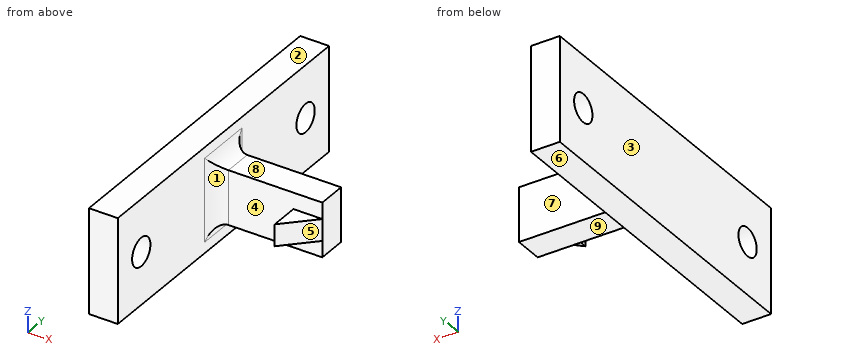
```python
from build123d import *

# Parameters (mm, degrees)
BOSS_EXTRUDE1_DEPTH      = 1
BOSS_EXTRUDE1_DEPTH_BACK = 1
SKETCH2_R                = 2
SKETCH2_R_2              = 1
BOSS_EXTRUDE2_DEPTH      = 4
SKETCH4_R                = 1.07
CUT_EXTRUDE1_DEPTH       = 233.583689314
BOSS_EXTRUDE3_DEPTH      = 2
SKETCH8_W                = 4
SKETCH8_H                = 8
BOSS_EXTRUDE4_DEPTH      = 2
CUT_EXTRUDE2_DEPTH       = 2
SKETCH10_W               = 16.5
SKETCH10_H               = 4
BOSS_EXTRUDE5_DEPTH      = 2.75
SKETCH11_W               = 16.5
SKETCH11_H               = 4
BOSS_EXTRUDE6_DEPTH      = 2.75
BOSS_EXTRUDE7_DEPTH      = 0.5
BOSS_EXTRUDE8_DEPTH      = 0.5
SKETCH14_W               = 1.779922348
SKETCH14_H               = 4
BOSS_EXTRUDE9_DEPTH      = 7.5
CUT_EXTRUDE3_DEPTH       = 10
CUT_EXTRUDE3_DEPTH_BACK  = 2
SKETCH15_W               = 40
SKETCH15_H               = 27.31360861
SKETCH16_W               = 14.5
SKETCH16_H               = 45
BOSS_EXTRUDE10_DEPTH     = 4
SKETCH18_R               = 1.95
CUT_EXTRUDE4_DEPTH       = 4
FILLET1_R                = 2


with BuildPart() as part:
    # Sketch2 → Boss-Extrude1 (new, two sides: drawn at the far end of the back side and taken through both)
    # profile 1 of 2: a face of its own
    with BuildSketch(Plane.XY.offset(-2.5).offset(-BOSS_EXTRUDE1_DEPTH_BACK)):
        with BuildLine():
            ThreePointArc((230.02407749, -2), (228.02407749, 0), (230.02407749, 2))
            Line((230.02407749, 2), (225.02407749, 2))
            Line((225.02407749, 2), (225.02407749, -2))
            Line((225.02407749, -2), (230.02407749, -2))
        make_face()
    # profile 2 of 2: a face of its own
    with BuildSketch(Plane.XY.offset(-2.5).offset(-BOSS_EXTRUDE1_DEPTH_BACK)):
        with Locations((230.02407749, 0)):
            Circle(SKETCH2_R)
        with Locations((230.02407749, 0)):
            Circle(SKETCH2_R_2, mode=Mode.SUBTRACT)
    extrude(amount=BOSS_EXTRUDE1_DEPTH + BOSS_EXTRUDE1_DEPTH_BACK)

    # Sketch3 → Boss-Extrude2 (add)
    with BuildSketch(Plane(origin=(0, 2, 0), x_dir=(1, 0, 0), z_dir=(0, 1, 0))):
        Polygon((223.02407749, 2.5), (225.02407749, 2.5), (225.02407749, 3.5), (222.02407749, 10.5), (216.095506061, 10.5), (216.095506061, 8.5), (221.095506061, 8.5), (223.02407749, 4), align=None)
        Polygon((222.02407749, -5.5), (225.02407749, 1.5), (225.02407749, 2.5), (223.02407749, 2.5), (223.02407749, 1), (221.095506061, -3.5), (216.095506061, -3.5), (216.095506061, -5.5), align=None)
    extrude(amount=-BOSS_EXTRUDE2_DEPTH)

    # Sketch4 → Cut-Extrude1 (cut, through all)
    with BuildSketch(Plane(origin=(0, 0, -10.5), x_dir=(-1, 0, 0), z_dir=(0, 0, -1))):
        with Locations((-218.095506061, 0)):
            Circle(SKETCH4_R)
    extrude(amount=-CUT_EXTRUDE1_DEPTH, mode=Mode.SUBTRACT)

    # Sketch6 → Boss-Extrude3 (add)
    with BuildSketch(Plane.XY.offset(-1.5)):
        Polygon((230.02407749, 2), (240.02407749, 2), (240.02407749, -2), (230.02407749, -2), (228.102487775, -2), (228.102487775, 2), align=None)
    extrude(amount=-BOSS_EXTRUDE3_DEPTH)

    # Sketch8 → Boss-Extrude4 (add)
    with BuildSketch(Plane(origin=(0, 0, -3.5), x_dir=(-1, 0, 0), z_dir=(0, 0, -1))):
        with Locations((-238.02407749, -2)):
            Rectangle(SKETCH8_W, SKETCH8_H)
    extrude(amount=-BOSS_EXTRUDE4_DEPTH)

    # Sketch9 → Cut-Extrude2 (cut)
    with BuildSketch(Plane(origin=(0, 0, -3.5), x_dir=(-1, 0, 0), z_dir=(0, 0, -1))):
        Polygon((-236.02407749, -6), (-240.02407749, -6), (-240.02407749, -2), align=None)
    extrude(amount=-CUT_EXTRUDE2_DEPTH, mode=Mode.SUBTRACT)

    # Sketch10 → Boss-Extrude5 (add)
    with BuildSketch(Plane(origin=(0, 0, -3.5), x_dir=(-1, 0, 0), z_dir=(0, 0, -1))):
        with Locations((-231.77407749, 0)):
            Rectangle(SKETCH10_W, SKETCH10_H)
    extrude(amount=BOSS_EXTRUDE5_DEPTH)

    # Sketch11 → Boss-Extrude6 (add)
    with BuildSketch(Plane.XY.offset(-1.5)):
        with Locations((231.77407749, 0)):
            Rectangle(SKETCH11_W, SKETCH11_H)
    extrude(amount=BOSS_EXTRUDE6_DEPTH)

    # Sketch12 → Boss-Extrude7 (add)
    with BuildSketch(Plane(origin=(0, 0, -3.5), x_dir=(-1, 0, 0), z_dir=(0, 0, -1))):
        Polygon((-240.02407749, -2), (-236.02407749, -6), (-236.02407749, -2), align=None)
    extrude(amount=BOSS_EXTRUDE7_DEPTH)

    # Sketch13 → Boss-Extrude8 (add)
    with BuildSketch(Plane.XY.offset(-1.5)):
        Polygon((236.02407749, -2), (236.02407749, -6), (240.02407749, -2), align=None)
    extrude(amount=BOSS_EXTRUDE8_DEPTH)

    # Sketch14 → Boss-Extrude9 (add)
    with BuildSketch(Plane(origin=(0, 0, -6.25), x_dir=(-1, 0, 0), z_dir=(0, 0, -1))):
        with Locations((-223.914038664, 0)):
            Rectangle(SKETCH14_W, SKETCH14_H)
    extrude(amount=-BOSS_EXTRUDE9_DEPTH)

    # Sketch15 → Cut-Extrude3 (cut, two sides: drawn at the far end of the back side and taken through both)
    with BuildSketch(Plane.ZY.offset(-223.02407749).offset(-CUT_EXTRUDE3_DEPTH_BACK)):
        with Locations((-2.5, 0)):
            Rectangle(SKETCH15_W, SKETCH15_H)
    extrude(amount=CUT_EXTRUDE3_DEPTH + CUT_EXTRUDE3_DEPTH_BACK, mode=Mode.SUBTRACT)

    # Sketch16 → Boss-Extrude10 (add)
    with BuildSketch(Plane.ZY.offset(-225.02407749)):
        with Locations((-2.5, 0)):
            Rectangle(SKETCH16_W, SKETCH16_H)
    extrude(amount=BOSS_EXTRUDE10_DEPTH)

    # Sketch18 → Cut-Extrude4 (cut)
    with BuildSketch(Plane.ZY.offset(-221.02407749)):
        with Locations((-2.5, 17.5)):
            Circle(SKETCH18_R)
        with Locations((-2.5, -17.5)):
            Circle(SKETCH18_R)
    extrude(amount=-CUT_EXTRUDE4_DEPTH, mode=Mode.SUBTRACT)

    # Fillet1
    fillet1_edges = [part.edges().sort_by_distance(p)[0] for p in [
        (225.02407749, 0, 1.25),
        (225.02407749, 0, -6.25),
        (225.02407749, -2, -2.5),
        (225.02407749, 2, -2.5),
    ]]
    fillet(fillet1_edges, radius=FILLET1_R)


solid = part.part
```
The model under review builds one solid part; all positions refer to its coordinate system, in mm. Face numbers are marked on the shaded views. A direction names the side the tool comes from. Round coordinates to 2 decimals unless told otherwise and drop trailing zeros. Write each loop counter-clockwise with the first axis right and the second up, starting at its lowest first coordinate (ties: lowest second). Pieces come first, ordered by that corner, then holes. Notation, with made-up numbers: (6, 80.5) -> (22, 80.5) arc R23 ccw to (22, 107.5) -> close; hole circle Ø8 at (82, -2.75). An arc over 180 degrees is marked (long way). Use CSV: the item, a comma, the result in double quotes.
Q1. To check wall thickness, follow probe 1 along Y at (x, z) = (223.1, -2.5); probe 2 along X at (y, z) = (-9.5, -6.75); probe 3 along Y at (x, z) = (231.5, -3.25). State the ranges of each line that lie inside material, in increasing order. Write a range as [from, to].
Checks:
probe 1,"[-22.5, -19.45], [-15.55, 15.55], [19.45, 22.5]"
probe 2,"[221.02, 225.02]"
probe 3,"[-2, 2]"
Q2. For the marked faces 5, 6, 7, 8 and 9, list the 3-axis set-ups (+Z, -Z, +X, -X, +Y, -Y) from which the entire face can be reached by the end or side of a thin tool; tool diameter is ignored.
Checks:
face 5,"+Z, -Z, +X, -Y"
face 6,"-Z, +X, -X, +Y, -Y"
face 7,"+Z, -Z, +X, +Y"
face 8,"+Z, +X, +Y, -Y"
face 9,"-Z, +X, +Y, -Y"
Q3. For pin 1 Ø4 at (x, z) = (232.5, -3) entering from -Y; pin 2 Ø3 at (x, y) = (231, -0.5) entering from -Z; pin 3 Ø4.5 at (y, z) = (17.5, -2.5) entering from +X, all flat-tipped, find the tip position at first contact; note any pin that passes through.
Checks:
pin 1,"y = -2"
pin 2,"z = -6.25"
pin 3,"x = 225.02"
Q4. Consider section B-B (z = -2.5). Give the boundary of the cut face in (x, y).
Checks:
outline,"(221.02, -22.5) -> (225.02, -22.5) -> (225.02, -19.45) -> (221.02, -19.45) -> close; (221.02, -15.55) -> (225.02, -15.55) -> (225.02, -4) arc R2 cw to (227.02, -2) -> (236.02, -2) -> (236.02, -6) -> (240.02, -2) -> (240.02, 2) -> (227.02, 2) arc R2 cw to (225.02, 4) -> (225.02, 15.55) -> (221.02, 15.55) -> close; (221.02, 19.45) -> (225.02, 19.45) -> (225.02, 22.5) -> (221.02, 22.5) -> close"
Q5. Consider section C-C (x = 224.25). Give the boundary of the cut face in (y, z), then the cut area to 3 significant figures.
Checks:
outline,"(-22.5, -9.75) -> (22.5, -9.75) -> (22.5, 4.75) -> (-22.5, 4.75) -> close; hole circle Ø3.9 at (-17.5, -2.5); hole circle Ø3.9 at (17.5, -2.5)"
area,"629 mm²"
Q6. Consider section A-A (y = 17.5). Give the boundary of the cut face in (x, z).
Checks:
outline,"(221.02, -9.75) -> (225.02, -9.75) -> (225.02, -4.45) -> (221.02, -4.45) -> close; (221.02, -0.55) -> (225.02, -0.55) -> (225.02, 4.75) -> (221.02, 4.75) -> close"
Q7. Consider section D-D (z = 4.25). Give the boundary of the cut face in (x, y), then the cut area to 3 significant figures.
Checks:
outline,"(221.02, -22.5) -> (225.02, -22.5) -> (225.02, 22.5) -> (221.02, 22.5) -> close"
area,"180 mm²"
Q8. Mouldability with a two-part tool opening along X and no side actions: class the marked faces 1, 2, 3 and 4 as released by +X, released by -X, zero draft, split by the parting line, or undercut.
Checks:
face 1,"undercut"
face 2,"zero draft"
face 3,"released by -X"
face 4,"undercut"
